from build123d import *

# Parameters (mm, degrees)
SKETCH1_R           = 1.5
BOSS_EXTRUDE1_DEPTH = 2


with BuildPart() as part:
    # Sketch1 → Boss-Extrude1 (new body)
    with BuildSketch(Plane.XY):
        Polygon((0, 370), (0, -370), (-14.226497308, -370), (-20, -360), (-14.226497308, -360), (-20, -350), (-14.226497308, -350), (-20, -340), (-14.226497308, -340), (-20, -330), (-14.226497308, -330), (-20, -320), (-14.226497308, -320), (-20, -310), (-14.226497308, -310), (-20, -300), (-14.226497308, -300), (-20, -290), (-14.226497308, -290), (-20, -280), (-14.226497308, -280), (-20, -270), (-14.226497308, -270), (-20, -260), (-14.226497308, -260), (-20, -250), (-14.226497308, -250), (-20, -240), (-14.226497308, -240), (-20, -230), (-14.226497308, -230), (-20, -220), (-14.226497308, -220), (-20, -210), (-14.226497308, -210), (-20, -200), (-14.226497308, -200), (-20, -190), (-14.226497308, -190), (-20, -180), (-14.226497308, -180), (-20, -170), (-14.226497308, -170), (-20, -160), (-14.226497308, -160), (-20, -150), (-14.226497308, -150), (-20, -140), (-14.226497308, -140), (-20, -130), (-14.226497308, -130), (-20, -120), (-14.226497308, -120), (-20, -110), (-14.226497308, -110), (-20, -100), (-14.226497308, -100), (-20, -90), (-14.226497308, -90), (-20, -80), (-14.226497308, -80), (-20, -70), (-14.226497308, -70), (-20, -60), (-14.226497308, -60), (-20, -50), (-14.226497308, -50), (-20, -40), (-14.226497308, -40), (-20, -30), (-14.226497308, -30), (-20, -20), (-14.226497308, -20), (-20, -10), (-14.226497308, -10), (-20, 0), (-14.226497308, 0), (-20, 10), (-14.226497308, 10), (-20, 20), (-14.226497308, 20), (-20, 30), (-14.226497308, 30), (-20, 40), (-14.226497308, 40), (-20, 50), (-14.226497308, 50), (-20, 60), (-14.226497308, 60), (-20, 70), (-14.226497308, 70), (-20, 80), (-14.226497308, 80), (-20, 90), (-14.226497308, 90), (-20, 100), (-14.226497308, 100), (-20, 110), (-14.226497308, 110), (-20, 120), (-14.226497308, 120), (-20, 130), (-14.226497308, 130), (-20, 140), (-14.226497308, 140), (-20, 150), (-14.226497308, 150), (-20, 160), (-14.226497308, 160), (-20, 170), (-14.226497308, 170), (-20, 180), (-14.226497308, 180), (-20, 190), (-14.226497308, 190), (-20, 200), (-14.226497308, 200), (-20, 210), (-14.226497308, 210), (-20, 220), (-14.226497308, 220), (-20, 230), (-14.226497308, 230), (-20, 240), (-14.226497308, 240), (-20, 250), (-14.226497308, 250), (-20, 260), (-14.226497308, 260), (-20, 270), (-14.226497308, 270), (-20, 280), (-14.226497308, 280), (-20, 290), (-14.226497308, 290), (-20, 300), (-14.226497308, 300), (-20, 310), (-14.226497308, 310), (-20, 320), (-14.226497308, 320), (-20, 330), (-14.226497308, 330), (-20, 340), (-14.226497308, 340), (-20, 350), (-14.226497308, 350), (-20, 360), (-14.226497308, 360), (-20, 370), align=None)
        with Locations((-8, 350)):
            Circle(SKETCH1_R, mode=Mode.SUBTRACT)
        with Locations((-8, 210)):
            Circle(SKETCH1_R, mode=Mode.SUBTRACT)
        with Locations((-8, 70)):
            Circle(SKETCH1_R, mode=Mode.SUBTRACT)
        with Locations((-8, -70)):
            Circle(SKETCH1_R, mode=Mode.SUBTRACT)
        with Locations((-8, -210)):
            Circle(SKETCH1_R, mode=Mode.SUBTRACT)
        with Locations((-8, -350)):
            Circle(SKETCH1_R, mode=Mode.SUBTRACT)
    extrude(amount=BOSS_EXTRUDE1_DEPTH)


solid = part.part
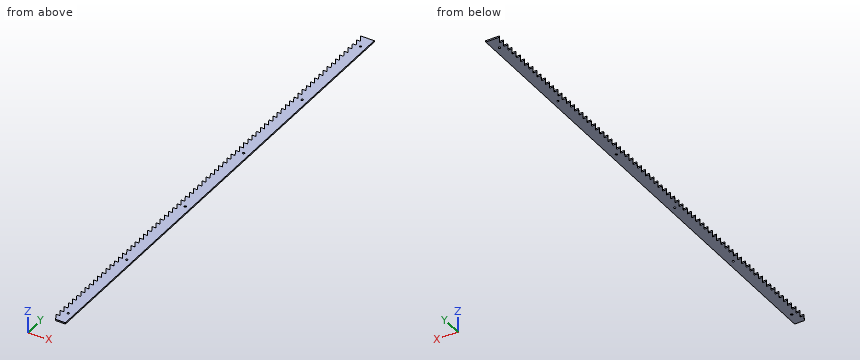
Build history of the part. All positions in model axes, mm. Coordinates: 2 decimals unless noted, no trailing zeros.
(1) Cut at A-A on z = 1.3. State how many separate pieces and enclosed holes the cut face has, and give its area (3 significant figures).
(2) Pin check, flat tip, straight feed: pin 1 Ø1 at (y, z) = (-136, 1) entering from -X. Stop position of the tip, or through.
(3) Drill centre lines: line 1 (X direction, y = -213.5, z = 0.4); line 2 (X direction, y = -52, z = 0.2). Where is each one in solid material? Low to high.
Working result:
1. separate pieces: 1
1. enclosed holes: 6
1. area: 12,600 mm2
2. pin 1: stops at x = -16.82
3. line 1: x = -17.98 to 0
3. line 2: x = -18.85 to 0
